For this review, take the finished solid that the model builds, in its own axes (mm). A direction names the side the tool comes from. Give positions to 0.01 mm unless a question says otherwise; leave off trailing zeros. Loops run counter-clockwise (first coordinate to the right, second up) from the corner with the lowest first, then second, coordinate; pieces in that order, holes last. Notation, with made-up numbers: (9, 78.5) - (64, 78.5) arc R28 ccw to (64, 114.5) - close; hole circle Ø11 at (32, 66). An arc over 180 degrees is marked (long way). Put each result on its own line as item: value.
from build123d import *

# Parameters (mm, degrees)
F0_W      = 95.1874652
F0_H      = 27.6999954
F0_R      = 6.7062477
F1_DEPTH  = 1.5875
F2_R      = 10.6749977
F3_R      = 7.5
F4_DEPTH  = 12
F5_DEPTH  = 4.7625
F6_R      = 1.7272
F6_R_2    = 3.175
F7_DEPTH  = 13.5875
F8_R      = 3.96875
F9_DEPTH  = 7.2375014
F11_DEPTH = 3.175


with BuildPart() as f1:
    # F0 (on Top) → F1 (new body)
    with BuildSketch(Plane.XY):
        with Locations((47.5937326, -13.8499977)):
            Rectangle(F0_W, F0_H)
        with Locations((10.6749977, -10.6749977)):
            Circle(F0_R, mode=Mode.SUBTRACT)
        with Locations((84.5124675, -10.6749977)):
            Circle(F0_R, mode=Mode.SUBTRACT)
    extrude(amount=F1_DEPTH)

    # F2
    f2_edges = [f1.edges().sort_by_distance(p)[0] for p in [
        (0, 0, 0.79375),
        (95.187465, 0, 0.79375),
    ]]
    fillet(f2_edges, radius=F2_R)

    # F3 (on face) → F4 (join)
    with BuildSketch(Plane.XY.offset(1.5875)):
        with BuildLine():
            Line((0, -10.6749977), (0, -21.3499954))
            Line((0, -21.3499954), (95.1874652, -21.3499954))
            Line((95.1874652, -21.3499954), (95.1874652, -10.6749977))
            ThreePointArc((95.1874652, -10.6749977), (92.0608307628, -3.1266344372), (84.5124675, 0))
            Line((84.5124675, 0), (10.6749977, 0))
            ThreePointArc((10.6749977, 0), (3.1266344372, -3.1266344372), (0, -10.6749977))
        make_face()
        with Locations((10.6749977, -10.6749977)):
            Circle(F3_R, mode=Mode.SUBTRACT)
        with Locations((84.5124675, -10.6749977)):
            Circle(F3_R, mode=Mode.SUBTRACT)
    extrude(amount=F4_DEPTH)

    # F5 (add): a face of the model
    f5_faces = [f1.faces().sort_by_distance(p)[0] for p in [
        (47.5937326, -24.5249954, 1.5875),
    ]]
    extrude(f5_faces, amount=F5_DEPTH)

    # F6 (on face) → F7 (cut, through all)
    with BuildSketch(Plane.XY.offset(13.5875)):
        with Locations((42.4937295646, -10.6749977)):
            Circle(F6_R)
        with Locations((71.4562175, -10.6749977)):
            Circle(F6_R)
        with Locations((32.1375151, -7.6956539)):
            Circle(F6_R_2)
    extrude(amount=-F7_DEPTH, mode=Mode.SUBTRACT)

    # F8 (on face) → F9 (cut)
    with BuildSketch(Plane(origin=(0, 0, 0), x_dir=(1, 0, 0), z_dir=(0, 0, -1))):
        with Locations((71.4562175, 10.6749977)):
            Circle(F8_R)
        with Locations((42.4937295646, 10.6749977)):
            Circle(F8_R)
    extrude(amount=-F9_DEPTH, mode=Mode.SUBTRACT)

    # F10 (on face) → F11 (cut)
    with BuildSketch(Plane.XY.offset(13.5875)):
        Polygon((34.7475158461, -3.175), (29.5275143539, -3.175), (26.9175136078, -7.6956539), (29.5275143539, -12.2163078), (34.7475158461, -12.2163078), (37.3575165922, -7.6956539), align=None)
    extrude(amount=-F11_DEPTH, mode=Mode.SUBTRACT)


solid = f1.part
1) Wall thickness on line 1 (X direction, y = -15.25, z = 5.25); line 2 (X direction, y = -17.25, z = 6); line 3 (X direction, y = -12, z = 11.5): over which ranges is each line inside the solid? List them lowest first.
Geometry check:
line 1: x = 0 to 4.73, 16.62 to 78.57, 90.46 to 95.19
line 2: x = 0 to 7.07, 14.28 to 80.9, 88.12 to 95.19
line 3: x = 0 to 3.29, 18.06 to 29.4, 34.87 to 41.39, 43.6 to 70.35, 72.56 to 77.13, 91.89 to 95.19
2) Take a section at B-B on x = 83.5. State the section outline as (y, z) points, and give its area (3 significant figures).
Geometry check:
outline: (-27.7, 0) - (-17.3, 0) - (-17.3, 1.59) - (-18.11, 1.59) - (-18.11, 13.59) - (-21.35, 13.59) - (-21.35, 6.35) - (-27.7, 6.35) - close; (-4.05, 0) - (0, 0) - (0, 13.59) - (-3.24, 13.59) - (-3.24, 1.59) - (-4.05, 1.59) - close
area: 131 mm²
3) Insertion check: pin 1 Ø2 at (x, z) = (60, 10) entering from -Y; pin 2 Ø16.5 at (x, y) = (86, -12) entering from +Z; pin 3 Ø3 at (x, y) = (42.49, -10.67) entering from +Z; pin 4 Ø4.5 at (x, y) = (34, -7.5) entering from +Z. Each pin has a flat end and moves straight along its axis. Give the tip position at first contact, or say it passes through.
Geometry check:
pin 1: stops at y = -21.35
pin 2: stops at z = 13.59
pin 3: passes through
pin 4: stops at z = 10.41
4) Take a section at C-C on y = -16.5. State the section outline as (x, z) points, and give its area (3 significant figures).
Geometry check:
outline: (0, 0) - (7.35, 0) - (7.35, 1.59) - (5.95, 1.59) - (5.95, 13.59) - (0, 13.59) - close; (14, 0) - (81.19, 0) - (81.19, 1.59) - (79.79, 1.59) - (79.79, 13.59) - (15.4, 13.59) - (15.4, 1.59) - (14, 1.59) - close; (87.84, 0) - (95.19, 0) - (95.19, 13.59) - (89.24, 13.59) - (89.24, 1.59) - (87.84, 1.59) - close
area: 1,050 mm²
5) For faces 1 (the face through (73.2, -9.8, 7.238)), 2 (the face through (47, -21.35, 10)), 3 (the face through (9.049, -17.997, 7.504)), list the 3-axis set-ups (+Z, -Z, +X, -X, +Y, -Y) from which the entire face can be reached by the end or side of a thin tool; tool diameter is ignored.
Geometry check:
face 1: -Z
face 2: +Z, +X, -X, -Y
face 3: +Z
6) Take a section at D-D on x = 66. State the section outline as (y, z) points.
Geometry check:
outline: (-27.7, 0) - (0, 0) - (0, 13.59) - (-21.35, 13.59) - (-21.35, 6.35) - (-27.7, 6.35) - close
7) Draft analysis for pull direction X (two halves, no side actions). For faces 4 (the face through (32, -12.216, 12)), 5 (the face through (95.187, -17, 7)), 6 (the face through (48, 0, 7)), state which applies: pulls with the +X half, pulls with the -X half, needs draft (parallel to the pull), parting line crosses it, or undercut.
Geometry check:
face 4: undercut
face 5: pulls with the +X half
face 6: needs draft
8) Take a section at A-A on z = 12. State the section outline as (x, y) points (3 decimals), and give its area (3 significant figures).
Geometry check:
outline: (0, -21.35) - (95.187, -21.35) - (95.187, -10.675) arc R10.675 ccw to (84.512, 0) - (10.675, 0) arc R10.675 ccw to (0, -10.675) - close; hole circle Ø15 at (10.675, -10.675); hole (26.918, -7.696) - (29.528, -12.216) - (34.748, -12.216) - (37.358, -7.696) - (34.748, -3.175) - (29.528, -3.175) - close; hole circle Ø3.454 at (42.494, -10.675); hole circle Ø3.454 at (71.456, -10.675); hole circle Ø15 at (84.512, -10.675)
area: 1,540 mm²
